from build123d import *

# Parameters (mm, degrees)
SKETCH_1_W      = 30.2
SKETCH_1_H      = 20.2
EXTRUDE_1_DEPTH = 10.2
FILLET_1_R      = 1
SKETCH_2_R      = 0.4
EXTRUDE_3_DEPTH = 4


with BuildPart() as part:
    # Эскиз1 → Бобышка-Вытянуть1 (new body)
    with BuildSketch(Plane(origin=(0, 0, 0), x_dir=(1, 0, 0), z_dir=(0, 1, 0))):
        Rectangle(SKETCH_1_W, SKETCH_1_H)
    extrude(amount=EXTRUDE_1_DEPTH)

    # Скругление1
    fillet_1_edges = [part.edges().sort_by_distance(p)[0] for p in [
        (-15.1, 10.2, 0),
        (0, 10.2, 10.1),
        (15.1, 10.2, 0),
        (0, 10.2, -10.1),
        (15.1, 5.1, 10.1),
        (-15.1, 5.1, 10.1),
        (-15.1, 5.1, -10.1),
        (15.1, 5.1, -10.1),
    ]]
    fillet(fillet_1_edges, radius=FILLET_1_R)

    # Эскиз2 → Бобышка-Вытянуть3 (add)
    with BuildSketch(Plane.XZ):
        with Locations(Location((11.53, 7.72, 0), (0, 0, 90))):
            Circle(SKETCH_2_R)
        with Locations(Location((13.15, 5.73, 0), (0, 0, 90))):
            Circle(SKETCH_2_R)
        with Locations(Location((8.99, 7.72, 0), (0, 0, 90))):
            Circle(SKETCH_2_R)
        with Locations(Location((6.45, -7.52, 0), (0, 0, 90))):
            Circle(SKETCH_2_R)
        with Locations(Location((-6.25, 7.72, 0), (0, 0, 90))):
            Circle(SKETCH_2_R)
        with Locations(Location((-11.33, 7.72, 0), (0, 0, 90))):
            Circle(SKETCH_2_R)
        with Locations(Location((-11.33, -7.52, 0), (0, 0, 90))):
            Circle(SKETCH_2_R)
        with Locations(Location((-6.25, -7.52, 0), (0, 0, 90))):
            Circle(SKETCH_2_R)
        with Locations(Location((8.99, -7.52, 0), (0, 0, 90))):
            Circle(SKETCH_2_R)
        with Locations(Location((11.53, -7.52, 0), (0, 0, 90))):
            Circle(SKETCH_2_R)
    extrude(amount=EXTRUDE_3_DEPTH)


solid = part.part
Can you work these out from the model? Positions are in its coordinate system, mm. A direction names the side the tool comes from. Coordinates: 2 decimals unless noted, no trailing zeros. Order: outer loops, then holes, each group sorted by start corner. A loop starts at its lowest first (then second) coordinate and runs counter-clockwise, first axis right, second up. Notation, with made-up numbers: (19.25, 2.5) - (42.25, 2.5) arc R23 cw to (42.25, 12.5) - close; hole circle Ø1 at (37.25, -7). An arc over 180 degrees is marked (long way). Answer as a JSON object with one key per item and string values. Group by question number.
Q1. We'd pull the mould along X, two halves only. Please class faces 1 (the face through (0, 10.2, 0)), 2 (the face through (14.799, 4.664, 9.815)), 3 (the face through (13, -2, 6.1)), 4 (the face through (-6.1, -1.97, 8.09)): +X half, -X half, draft (parallel to the pull), parting line (faces both ways), or undercut.
Q2. Will this pin go through, and if not, where does the flat tip stop? P1, Ø1, axis at x = 7, z = -5.5, coming from the -Y side.
Q3. I need wall thicknesses on line 1 (Z direction, x = 6.5, y = -2); line 2 (Y direction, x = -11, z = -3.75); line 3 (Z direction, x = -13, y = 9.25). Which ranges of each line are inside material? Lowest first, please. Write a range as from..to.
Q4. Imagine slicing it at D-D (z = 7.72). Please give me the cut outline in (x, y), and give its area (3 significant figures).
Q5. On a 3-axis mill with a long thin cutter (end or side, diameter ignored), from which of +Z, -Z, +X, -X, +Y, -Y can I reach the whole of each face in a straight line? I mean faces 5 (the face through (-14.815, 9.899, -0.127)), 6 (the face through (6.6, -1.97, -7.15)). Say none if no direction works.
Q6. Imagine slicing it at A-A (y = -0.5). Give the number of separate pieces and of enclosed holes in the cut face, and give its area (3 significant figures).
Q7. Imagine slicing it at C-C (x = 13.15). Please give me the cut outline in (y, z).
Q8. Imagine slicing it at B-B (z = -7.52). Please give me the cut outline in (x, y), and give its area (3 significant figures).
Determined:
{
 "1": {"face 1": "draft", "face 2": "+X half", "face 3": "parting line", "face 4": "undercut"},
 "2": {"P1": "stops at y = 0"},
 "3": {"line 1": "z = -7.92..-7.12", "line 2": "y = 0..10.2", "line 3": "z = -10.1..10.1"},
 "4": {"outline": "(-15.1, 0) - (-11.73, 0) - (-11.73, -4) - (-10.93, -4) - (-10.93, 0) - (-6.65, 0) - (-6.65, -4) - (-5.85, -4) - (-5.85, 0) - (8.59, 0) - (8.59, -4) - (9.39, -4) - (9.39, 0) - (11.13, 0) - (11.13, -4) - (11.93, -4) - (11.93, 0) - (15.1, 0) - (15.1, 9.2) arc R1 ccw to (14.1, 10.2) - (-14.1, 10.2) arc R1 ccw to (-15.1, 9.2) - close", "area": "320 mm2"},
 "5": {"face 5": "+Z, -Z, -X, +Y", "face 6": "-Y"},
 "6": {"separate pieces": "10", "enclosed holes": "0", "area": "5.03 mm2"},
 "7": {"outline": "(-4, 5.33) - (0, 5.33) - (0, -10.1) - (9.2, -10.1) arc R1 ccw to (10.2, -9.1) - (10.2, 9.1) arc R1 ccw to (9.2, 10.1) - (0, 10.1) - (0, 6.13) - (-4, 6.13) - close"},
 "8": {"outline": "(-15.1, 0) - (-11.73, 0) - (-11.73, -4) - (-10.93, -4) - (-10.93, 0) - (-6.65, 0) - (-6.65, -4) - (-5.85, -4) - (-5.85, 0) - (6.05, 0) - (6.05, -4) - (6.85, -4) - (6.85, 0) - (8.59, 0) - (8.59, -4) - (9.39, -4) - (9.39, 0) - (11.13, 0) - (11.13, -4) - (11.93, -4) - (11.93, 0) - (15.1, 0) - (15.1, 9.2) arc R1 ccw to (14.1, 10.2) - (-14.1, 10.2) arc R1 ccw to (-15.1, 9.2) - close", "area": "324 mm2"}
}
